from build123d import *

# Parameters (mm, degrees)
SKETCH1_R                = 1.5875
BOSS_EXTRUDE1_DEPTH      = 21.89226
SKETCH2_R                = 1.19126
BOSS_EXTRUDE2_DEPTH      = 0.381
SKETCH3_R                = 1.5875
BOSS_EXTRUDE3_DEPTH      = 1.27
CHAMFER1_SIZE            = 0.381
CHAMFER1_OF_MIRROR1_SIZE = 0.381


with BuildPart() as part:
    # Sketch1 → Boss-Extrude1 (new body, symmetric)
    with BuildSketch(Plane.XY):
        Circle(SKETCH1_R)
    extrude(amount=BOSS_EXTRUDE1_DEPTH, both=True)

    # Sketch2 → Boss-Extrude2 (add)
    with BuildSketch(Plane.XY.offset(21.89226)):
        Circle(SKETCH2_R)
    boss_extrude2 = extrude(amount=BOSS_EXTRUDE2_DEPTH)

    # Sketch3 → Boss-Extrude3 (add)
    with BuildSketch(Plane.XY.offset(22.27326)):
        Circle(SKETCH3_R)
    boss_extrude3 = extrude(amount=BOSS_EXTRUDE3_DEPTH)

    # Chamfer1
    chamfer1_edges = [part.edges().sort_by_distance(p)[0] for p in [
        (-1.5875, 0, 23.54326),
    ]]
    chamfer(chamfer1_edges, length=CHAMFER1_SIZE)

    # Mirror1: Boss-Extrude2, Boss-Extrude3 across plane
    add(boss_extrude2.mirror(Plane.XY))
    add(boss_extrude3.mirror(Plane.XY))

    # Chamfer1 of Mirror1
    chamfer1_of_mirror1_edges = [part.edges().sort_by_distance(p)[0] for p in [
        (-1.5875, 0, -23.54326),
    ]]
    chamfer(chamfer1_of_mirror1_edges, length=CHAMFER1_OF_MIRROR1_SIZE)


solid = part.part
Could you check a few things on this model? Use its own coordinates, in mm. A direction names the side the tool comes from. Round coordinates to 2 decimals unless told otherwise and drop trailing zeros. Order: outer loops, then holes, each group sorted by start corner. A loop starts at its lowest first (then second) coordinate and runs counter-clockwise, first axis right, second up.
Q1. Please list where these lines run through material, in increasing order: probe 1 along Z at (x, y) = (1.2, 0.4); probe 2 along Z at (x, y) = (-1.3, 0.6); probe 3 along Y at (x, z) = (-0.1, -3).
Geometry says:
probe 1: z = -23.48 to -22.27, -21.89 to 21.89, 22.27 to 23.48
probe 2: z = -23.32 to -22.27, -21.89 to 21.89, 22.27 to 23.32
probe 3: y = -1.58 to 1.58
Q2. Imagine slicing it at A-A, the plane z = -3. List the corners of the cut face in (x, y) for me (1 decimal).
Geometry says:
outline: circle Ø3.2 at (0, 0)
Q3. I'm going to push a flat-ended pin straight in: P1, Ø1, axis at x = 1, z = 12.5, coming from the +Y side. Where does the tip first touch, or does it pass through?
Geometry says:
P1: stops at y = 1.51
Q4. Which directions (+Z, -Z, +X, -X, +Y, -Y) give clear straight access to the entire face, cutting with the end or side of a thin tool? Please do faces 1 (the face through (1, 1, -21.892)), 2 (the face through (-0.34, -1.55, 0.31)).
Geometry says:
face 1: none
face 2: +Z, -Z
